Check sheet for the modelled part. Datum: model origin and axes. Units: mm. A direction names the side the tool comes from. Round coordinates to 2 decimals unless told otherwise and drop trailing zeros. Write each loop counter-clockwise with the first axis right and the second up, starting at its lowest first coordinate (ties: lowest second). Pieces come first, ordered by that corner, then holes. Notation, with made-up numbers: (-35.75, -19) -> (-11.75, -19) arc R29 cw to (-11.75, 16) -> close; hole circle Ø10 at (22.25, 22.25). An arc over 180 degrees is marked (long way). One line per item, written item: value.
from build123d import *

# Parameters (mm, degrees)
SKETCH1_W            = 40
SKETCH1_H            = 76
BOSS_EXTRUDE1_DEPTH  = 10
SKETCH2_W            = 40
SKETCH2_H            = 76
SKETCH2_W_2          = 30
SKETCH2_H_2          = 60
BOSS_EXTRUDE2_DEPTH  = 40
SKETCH3_W            = 25
SKETCH3_H            = 30
CUT_EXTRUDE1_DEPTH   = 100.37806599
SKETCH4_W            = 60
SKETCH4_H            = 30
CUT_EXTRUDE2_DEPTH   = 100.37806599
SKETCH9_R            = 1.778
SKETCH9_R_2          = 1.778000002
CUT_EXTRUDE4_DEPTH   = 40
BOSS_EXTRUDE4_START  = -10
SKETCH12_R           = 1.778
BOSS_EXTRUDE4_DEPTH  = 10
SKETCH13_W           = 40
SKETCH13_H           = 10
BOSS_EXTRUDE5_DEPTH  = 7
SKETCH14_W           = 40
SKETCH14_H           = 10
BOSS_EXTRUDE6_DEPTH  = 7
SKETCH16_W           = 40
SKETCH16_H           = 7
BOSS_EXTRUDE7_DEPTH  = 4.5
SKETCH17_W           = 40
SKETCH17_H           = 4.5
BOSS_EXTRUDE8_DEPTH  = 14
SKETCH18_W           = 40
SKETCH18_H           = 4.5
BOSS_EXTRUDE9_DEPTH  = 14
SKETCH19_W           = 40
SKETCH19_H           = 19
BOSS_EXTRUDE10_DEPTH = 2
BOSS_EXTRUDE11_DEPTH = 9
CUT_EXTRUDE6_START   = -7.5
SKETCH21_W           = 9
SKETCH21_H           = 10
CUT_EXTRUDE6_DEPTH   = 7.5
BOSS_EXTRUDE13_DEPTH = 2
CUT_EXTRUDE7_START   = -49
SKETCH25_W           = 2
SKETCH25_H           = 64
CUT_EXTRUDE7_DEPTH   = 49
SKETCH26_W           = 2
SKETCH26_H           = 64
CUT_EXTRUDE8_DEPTH   = 42
SKETCH27_W           = 60
SKETCH27_H           = 10
CUT_EXTRUDE10_DEPTH  = 10
SKETCH28_W           = 32.101148564
SKETCH28_H           = 16
BOSS_EXTRUDE14_DEPTH = 24
SKETCH29_W           = 32.101148564
SKETCH29_H           = 14
BOSS_EXTRUDE15_DEPTH = 4
SKETCH30_R           = 4.25
CUT_EXTRUDE11_DEPTH  = 2.5


with BuildPart() as part:
    # Sketch1 → Boss-Extrude1 (new body)
    with BuildSketch(Plane(origin=(0, 0, 0), x_dir=(1, 0, 0), z_dir=(0, 1, 0))):
        with Locations((20, 38)):
            Rectangle(SKETCH1_W, SKETCH1_H)
    extrude(amount=BOSS_EXTRUDE1_DEPTH)

    # Sketch2 → Boss-Extrude2 (add)
    with BuildSketch(Plane(origin=(0, 10, 0), x_dir=(1, 0, 0), z_dir=(0, 1, 0))):
        with Locations((20, 38)):
            Rectangle(SKETCH2_W, SKETCH2_H)
        with Locations((20, 38)):
            Rectangle(SKETCH2_W_2, SKETCH2_H_2, mode=Mode.SUBTRACT)
    extrude(amount=BOSS_EXTRUDE2_DEPTH)

    # Sketch3 → Cut-Extrude1 (cut, through all)
    with BuildSketch(Plane.XY):
        with Locations((20, 25)):
            Rectangle(SKETCH3_W, SKETCH3_H)
    extrude(amount=-CUT_EXTRUDE1_DEPTH, mode=Mode.SUBTRACT)

    # Sketch4 → Cut-Extrude2 (cut, through all)
    with BuildSketch(Plane.ZY):
        with Locations((-38, 25)):
            Rectangle(SKETCH4_W, SKETCH4_H)
    extrude(amount=-CUT_EXTRUDE2_DEPTH, mode=Mode.SUBTRACT)

    # Sketch9 → Cut-Extrude4 (cut)
    with BuildSketch(Plane.XZ):
        with Locations(Location((26.914797213, -38.414797213, 0), (0, 0, 270))):
            Circle(SKETCH9_R)
        with Locations(Location((13.085202787, -24.585202787, 0), (0, 0, 270))):
            Circle(SKETCH9_R)
        with Locations(Location((26.914797213, -24.585202787, 0), (0, 0, 270))):
            Circle(SKETCH9_R)
        with Locations(Location((29.778999999, -31.5, 0), (0, 0, 270))):
            Circle(SKETCH9_R)
        with Locations(Location((13.085202787, -38.414797213, 0), (0, 0, 270))):
            Circle(SKETCH9_R_2)
    extrude(amount=-CUT_EXTRUDE4_DEPTH, mode=Mode.SUBTRACT)

    # Sketch12 → Boss-Extrude4 (add)
    with BuildSketch(Plane(origin=(0, 10, 0), x_dir=(1, 0, 0), z_dir=(0, 1, 0)).offset(BOSS_EXTRUDE4_START)):
        with Locations((29.778999999, 31.5)):
            Circle(SKETCH12_R)
    extrude(amount=BOSS_EXTRUDE4_DEPTH)

    # Sketch13 → Boss-Extrude5 (add)
    with BuildSketch(Plane.XY):
        with Locations((20, 45)):
            Rectangle(SKETCH13_W, SKETCH13_H)
    extrude(amount=BOSS_EXTRUDE5_DEPTH)

    # Sketch14 → Boss-Extrude6 (add)
    with BuildSketch(Plane(origin=(0, 0, -76), x_dir=(-1, 0, 0), z_dir=(0, 0, -1))):
        with Locations((-20, 45)):
            Rectangle(SKETCH14_W, SKETCH14_H)
    extrude(amount=BOSS_EXTRUDE6_DEPTH)

    # Sketch16 → Boss-Extrude7 (add)
    with BuildSketch(Plane(origin=(0, 50, 0), x_dir=(1, 0, 0), z_dir=(0, 1, 0))):
        with Locations((20, 79.5)):
            Rectangle(SKETCH16_W, SKETCH16_H)
        with Locations((20, -3.5)):
            Rectangle(SKETCH16_W, SKETCH16_H)
    extrude(amount=BOSS_EXTRUDE7_DEPTH)

    # Sketch17 → Boss-Extrude8 (add)
    with BuildSketch(Plane(origin=(0, 0, -83), x_dir=(-1, 0, 0), z_dir=(0, 0, -1))):
        with Locations((-20, 56.75)):
            Rectangle(SKETCH17_W, SKETCH17_H)
    extrude(amount=-BOSS_EXTRUDE8_DEPTH)

    # Sketch18 → Boss-Extrude9 (add)
    with BuildSketch(Plane.XY.offset(7)):
        with Locations((20, 56.75)):
            Rectangle(SKETCH18_W, SKETCH18_H)
    extrude(amount=-BOSS_EXTRUDE9_DEPTH)

    # Sketch19 → Boss-Extrude10 (add)
    with BuildSketch(Plane(origin=(0, 0, -83), x_dir=(-1, 0, 0), z_dir=(0, 0, -1))):
        with Locations((-20, 49.5)):
            Rectangle(SKETCH19_W, SKETCH19_H)
    extrude(amount=BOSS_EXTRUDE10_DEPTH)

    # Sketch20 → Boss-Extrude11 (add)
    with BuildSketch(Plane(origin=(0, 0, -76), x_dir=(-1, 0, 0), z_dir=(0, 0, -1))):
        Polygon((0, 40), (0, 0), (-40, 0), (-40, 40), (-32.5, 40), (-32.5, 10), (-7.5, 10), (-7.5, 40), align=None)
    extrude(amount=BOSS_EXTRUDE11_DEPTH)

    # Sketch21 → Cut-Extrude6 (cut)
    with BuildSketch(Plane.ZY.offset(CUT_EXTRUDE6_START)):
        with Locations((-72.5, 15)):
            Rectangle(SKETCH21_W, SKETCH21_H)
    extrude(amount=CUT_EXTRUDE6_DEPTH, mode=Mode.SUBTRACT)

    # Sketch23 → Boss-Extrude13 (add)
    with BuildSketch(Plane.ZY):
        Polygon((-69, 59), (-69, 54.5), (-76, 54.5), (-76, 50), (0, 50), (0, 54.5), (-7, 54.5), (-7, 59), (7, 59), (7, 40), (0, 40), (0, 0), (-85, 0), (-85, 59), align=None)
        Polygon((-68, 40), (-68, 20), (-77, 20), (-77, 10), (-76.5, 10), (-8, 10), (-8, 40), align=None, mode=Mode.SUBTRACT)
    extrude(amount=BOSS_EXTRUDE13_DEPTH)

    # Sketch25 → Cut-Extrude7 (cut)
    with BuildSketch(Plane(origin=(0, 59, 0), x_dir=(1, 0, 0), z_dir=(0, 1, 0)).offset(CUT_EXTRUDE7_START)):
        with Locations((4, 38)):
            Rectangle(SKETCH25_W, SKETCH25_H)
    extrude(amount=CUT_EXTRUDE7_DEPTH, mode=Mode.SUBTRACT)

    # Sketch26 → Cut-Extrude8 (cut)
    with BuildSketch(Plane(origin=(0, 50, 0), x_dir=(1, 0, 0), z_dir=(0, 1, 0))):
        with Locations((4, 38)):
            Rectangle(SKETCH26_W, SKETCH26_H)
    extrude(amount=-CUT_EXTRUDE8_DEPTH, mode=Mode.SUBTRACT)

    # Sketch27 → Cut-Extrude10 (cut)
    with BuildSketch(Plane.ZY.offset(2)):
        with Locations((-38, 45)):
            Rectangle(SKETCH27_W, SKETCH27_H)
    extrude(amount=-CUT_EXTRUDE10_DEPTH, mode=Mode.SUBTRACT)

    # Sketch28 → Boss-Extrude14 (add)
    with BuildSketch(Plane(origin=(0, 59, 0), x_dir=(1, 0, 0), z_dir=(0, 1, 0))):
        with Locations((23.949425718, 77)):
            Rectangle(SKETCH28_W, SKETCH28_H)
    extrude(amount=BOSS_EXTRUDE14_DEPTH)

    # Sketch29 → Boss-Extrude15 (add)
    with BuildSketch(Plane(origin=(0, 59, 0), x_dir=(1, 0, 0), z_dir=(0, 1, 0))):
        with Locations((23.949425718, 0)):
            Rectangle(SKETCH29_W, SKETCH29_H)
    extrude(amount=BOSS_EXTRUDE15_DEPTH)

    # Sketch30 → Cut-Extrude11 (cut)
    with BuildSketch(Plane(origin=(0, 10, 0), x_dir=(1, 0, 0), z_dir=(0, 1, 0))):
        with Locations(Location((13.085202787, 24.585202787, 0), (0, 0, 270))):
            Circle(SKETCH30_R)
        with Locations(Location((13.085202787, 38.414797213, 0), (0, 0, 270))):
            Circle(SKETCH30_R)
        with Locations(Location((26.914797213, 38.414797213, 0), (0, 0, 270))):
            Circle(SKETCH30_R)
        with Locations(Location((26.914797213, 24.585202787, 0), (0, 0, 270))):
            Circle(SKETCH30_R)
    extrude(amount=-CUT_EXTRUDE11_DEPTH, mode=Mode.SUBTRACT)


solid = part.part
Item 1: Sectioned sample at D-D (x = 37). Enter the section's corners in (y, z), then the cut area to 3 significant figures.
Result set:
outline: (0, -85) -> (83, -85) -> (83, -69) -> (54.5, -69) -> (54.5, -76) -> (50, -76) -> (50, 0) -> (54.5, 0) -> (54.5, -7) -> (63, -7) -> (63, 7) -> (40, 7) -> (40, 0) -> (0, 0) -> close; hole (10, -68) -> (40, -68) -> (40, -8) -> (10, -8) -> close
area: 3,170 mm^2
Item 2: Sectioned sample at B-B (z = -72.5). Enter the section's corners in (x, y), then the cut area to 3 significant figures.
Result set:
outline: (-2, 0) -> (40, 0) -> (40, 50) -> (-2, 50) -> (-2, 20) -> (7.5, 20) -> (7.5, 40) -> (32.5, 40) -> (32.5, 10) -> (-2, 10) -> close; (-2, 54.5) -> (40, 54.5) -> (40, 83) -> (7.9, 83) -> (7.9, 59) -> (-2, 59) -> close
area: 2,210 mm^2
Item 3: Release check for a two-part mould opening along X. For faces 6 (the flat face through (20, 40, -76)), 7 (the flat face through (40, 41, -49)), 8 (the flat face through (22, 69, -69)) record: pulls with the +X half, pulls with the -X half, needs draft (parallel to the pull), parting line crosses it, or undercut.
Result set:
face 6: undercut
face 7: pulls with the +X half
face 8: needs draft
Item 4: Tool access check on faces 1 (the flat face through (19, 10, -42)), 2 (the flat face through (7.5, 25, -4)), 3 (the flat face through (3, 59, 0)), 4 (the flat face through (0, 30, -8)), 5 (the flat face through (4, 57, -6)). Record the directions out of +Z, -Z, +X, -X, +Y, -Y that give a thin tool (end or side, any length) a straight path to the whole face; none if there is none.
Result set:
face 1: none
face 2: +Z, -Z
face 3: +Z, -Z, -X, +Y
face 4: -X, +Y
face 5: +Y
Item 5: Sectioned sample at A-A (y = 33.5). Enter the section's corners in (x, z).
Result set:
outline: (-2, -85) -> (7.5, -85) -> (7.5, -68) -> (5, -68) -> (5, -70) -> (3, -70) -> (3, -68) -> (-2, -68) -> close; (-2, -8) -> (3, -8) -> (3, -6) -> (5, -6) -> (5, -8) -> (7.5, -8) -> (7.5, 0) -> (-2, 0) -> close; (32.5, -85) -> (40, -85) -> (40, -68) -> (32.5, -68) -> close; (32.5, -8) -> (40, -8) -> (40, 0) -> (32.5, 0) -> close
Item 6: Sectioned sample at C-C (y = 61.5). Enter the section's corners in (x, z).
Result set:
outline: (7.9, -85) -> (40, -85) -> (40, -69) -> (7.9, -69) -> close; (7.9, -7) -> (40, -7) -> (40, 7) -> (7.9, 7) -> close
Item 7: Depth check by flat-ended pin: pin 1 (17.5 mm diameter, centred on x = 30.5, y = 29.5, fed in from +Z); pin 2 (3 mm diameter, centred on x = 26.91, z = -38.41, fed in from -Y); pin 3 (14 mm diameter, centred on x = 22.5, y = 76, fed in from +Z); pin 4 (7 mm diameter, centred on x = 11.5, z = -24, fed in from +Y). Enter the tip coordinate at first touch or a pass-through.
Result set:
pin 1: z = 0
pin 2: through
pin 3: z = -69
pin 4: y = 10
Item 8: Material ranges on line 1 along Y through (x, z) = (27.5, -70); line 2 along Y through (x, z) = (21, -3.5); line 3 along Z through (x, y) = (4, 29), recorded low to high.
Result set:
line 1: 0 to 10, 40 to 50, 54.5 to 83
line 2: 0 to 10, 40 to 50, 54.5 to 63
line 3: -85 to -70, -6 to 0
